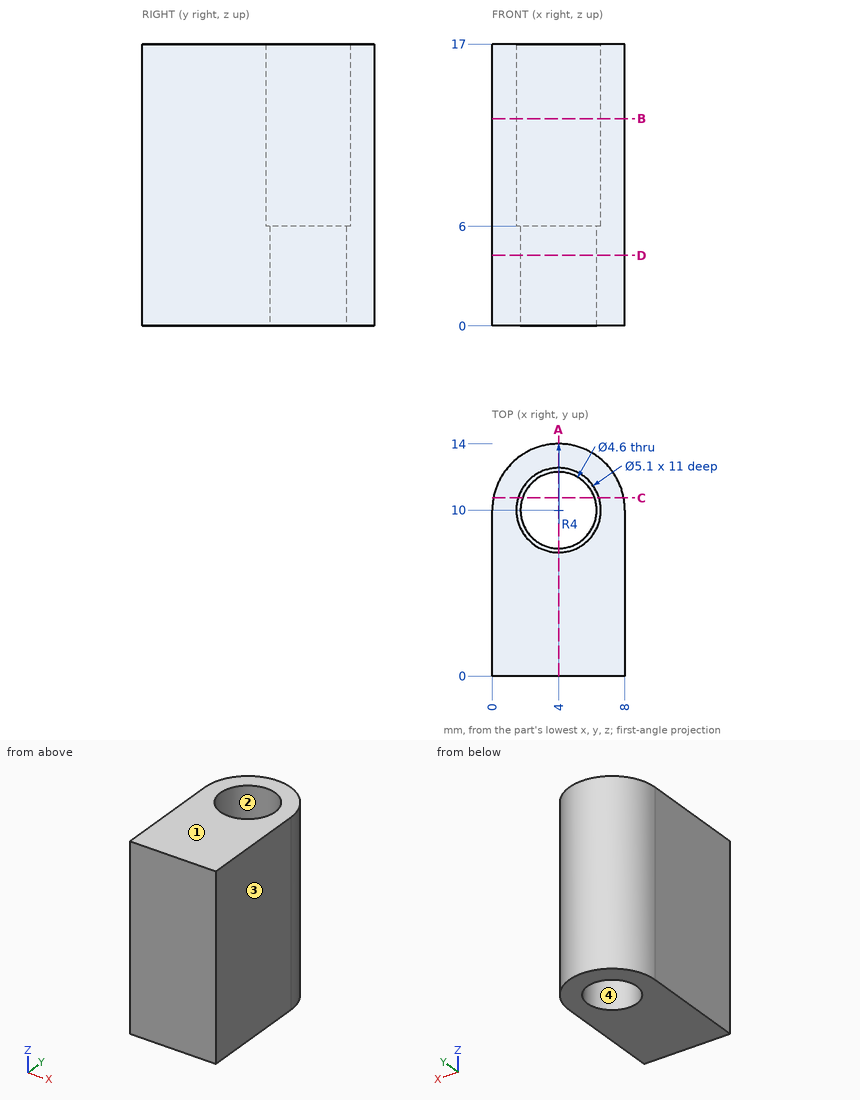
Here's the drawing with two shaded views (mm, measured from the low corner). I have some questions. Give positions to 0.01 mm unless a question says otherwise; leave off trailing zeros. Loops run counter-clockwise (first coordinate to the right, second up) from the corner with the lowest first, then second, coordinate; pieces in that order, holes last. Notation, with made-up numbers: M 27.5,-28.5 L 59.5,-28.5 A8 ccw 59.5,-23.5 Z; hole C 19,-30.5 d5. An arc over 180 degrees is marked long. Use one line per item in the form item = value. Start each with the question number.
Q1. If we section it at B-B (z = 12.5): Write out the boundary of the cut face in (x, y), then the cut area to 3 significant figures.
Q2. If we section it at A-A (x = 4): Write out the boundary of the cut face in (y, z), then the cut area to 3 significant figures.
Q3. If we section it at C-C (y = 10.75): Write out the boundary of the cut face in (x, z).
Q4. Thinking about a two-plate mould opening in X: for the marked faces 1, 2, 3 and 4, which applies, +X half, -X half, draft (parallel to the pull), parting line (faces both ways), or undercut?
Q5. Will these pins go through, and if not, where does the flat tip stop? pin 1 Ø5 at (y, z) = (4, 6) entering from -X; pin 2 Ø3 at (x, y) = (4, 10) entering from +Z; pin 3 Ø4 at (x, z) = (1.5, 13) entering from +Y.
Q6. If we section it at D-D (z = 4.25): Write out the boundary of the cut face in (x, y), then the cut area to 3 significant figures.
Q7. I need wall thicknesses on line 1 along Y through (x, z) = (4, 13.5); line 2 along Y through (x, z) = (4, 3); line 3 along X through (y, z) = (11, 10). Which ranges of each line are inside material? Lowest first, please.
Taken from the geometry:
q1.outline = M 0,0 L 8,0 L 8,10 A4 ccw 0,10 Z; hole C 4,10 d5.1
q1.area = 84.7 mm^2
q2.outline = M 0,0 L 7.7,0 L 7.7,6 L 7.45,6 L 7.45,17 L 0,17 Z; M 12.3,0 L 14,0 L 14,17 L 12.55,17 L 12.55,6 L 12.3,6 Z
q2.area = 154 mm^2
q3.outline = M 0.07,0 L 1.83,0 L 1.83,6 L 1.56,6 L 1.56,17 L 0.07,17 Z; M 6.17,0 L 7.93,0 L 7.93,17 L 6.44,17 L 6.44,6 L 6.17,6 Z
q4.face_1 = draft
q4.face_2 = undercut
q4.face_3 = +X half
q4.face_4 = undercut
q5.pin_1 = 0
q5.pin_2 = through
q5.pin_3 = 13.97
q6.outline = M 0,0 L 8,0 L 8,10 A4 ccw 0,10 Z; hole C 4,10 d4.6
q6.area = 88.5 mm^2
q7.line_1 = 0 to 7.45, 12.55 to 14
q7.line_2 = 0 to 7.7, 12.3 to 14
q7.line_3 = 0.13 to 1.65, 6.35 to 7.87
